```python
from build123d import *

# Parameters (mm, degrees)
F0_R      = 2.5
F1_DEPTH  = 85
F3_DEPTH  = 2.5
F5_DEPTH  = 25
F8_DEPTH  = 25
F9_DEPTH  = 25
F11_DEPTH = 25
F14_DEPTH = 102
F16_REACH = 96.5783545855
F18_REACH = 97.7333268634
F19_W     = 5
F19_H     = 41.5
F20_DEPTH = 25


with BuildPart() as f1:
    # F0 (on Front) → F1 (new body)
    with BuildSketch(Plane.XZ):
        Circle(F0_R)
    extrude(amount=F1_DEPTH)

    # F2 (on Right) → F3 (join, symmetric)
    with BuildSketch(Plane.YZ):
        Polygon((-69, 0), (-16, 0), (-22.4278760969, 7.6604444312), (-62.5721239031, 7.6604444312), align=None)
    extrude(amount=F3_DEPTH, both=True)

    # F4 (on face) → F5 (cut)
    with BuildSketch(Plane(origin=(-2.5, 0, 0), x_dir=(0, -1, 0), z_dir=(-1, 0, 0))):
        Polygon((56.5, 3), (53.5, 3), (50.5, 3), (44.1691353238, -4.5448307221), (62.8308646762, -4.5448307221), align=None)
        Polygon((40.8308646762, -4.5448307221), (34.5, 3), (31.5, 3), (28.5, 3), (22.1691353238, -4.5448307221), align=None)
    extrude(amount=-F5_DEPTH, mode=Mode.SUBTRACT)

    # F7 (on face) → F8 (cut)
    with BuildSketch(Plane(origin=(-2.5, 0, 0), x_dir=(0, -1, 0), z_dir=(-1, 0, 0))):
        Polygon((19.9172031134, 7.5), (22.2932472338, 7.5), (22.4278760969, 7.6604444312), (62.5721239031, 7.6604444312), (62.7067527662, 7.5), (66.5233954787, 7.5), (66.5233954787, 10.3880958632), (19.9172031134, 10.3880958632), align=None)
    extrude(amount=-F8_DEPTH, mode=Mode.SUBTRACT)

    # F6 (on face) → F9 (cut)
    with BuildSketch(Plane(origin=(0, 0, 3), x_dir=(1, 0, 0), z_dir=(0, 0, -1))):
        with BuildLine():
            ThreePointArc((1.45, 53.5), (1.0253048327, 54.5253048327), (0, 54.95))
            Line((0, 54.95), (0, 52.05))
            ThreePointArc((0, 52.05), (1.0253048327, 52.4746951673), (1.45, 53.5))
        make_face()
        with BuildLine():
            Line((0, 52.05), (0, 54.95))
            ThreePointArc((0, 54.95), (-1.45, 53.5), (0, 52.05))
        make_face()
    extrude(amount=-F9_DEPTH, mode=Mode.SUBTRACT)

    # F10 (on face) → F11 (cut)
    with BuildSketch(Plane(origin=(0, 0, 3), x_dir=(1, 0, 0), z_dir=(0, 0, -1))):
        with BuildLine():
            ThreePointArc((1.45, 31.5), (1.0253048327, 32.5253048327), (0, 32.95))
            Line((0, 32.95), (0, 30.05))
            ThreePointArc((0, 30.05), (1.0253048327, 30.4746951673), (1.45, 31.5))
        make_face()
        with BuildLine():
            Line((0, 30.05), (0, 32.95))
            ThreePointArc((0, 32.95), (-1.45, 31.5), (0, 30.05))
        make_face()
    extrude(amount=-F11_DEPTH, mode=Mode.SUBTRACT)

    # F13 (on face) → F14 (cut)
    with BuildSketch(Plane.XZ.offset(85)):
        with BuildLine():
            ThreePointArc((2.4, 0), (0, -2.4), (-2.4, 0))
            Line((-2.4, 0), (-2.4, 9.7710704431))
            Line((-2.4, 9.7710704431), (-6.1972029507, 9.7710704431))
            Line((-6.1972029507, 9.7710704431), (-6.1972029507, -5.7614380494))
            Line((-6.1972029507, -5.7614380494), (5.5722752586, -5.7614380494))
            Line((5.5722752586, -5.7614380494), (5.5722752586, 8.8547384366))
            Line((5.5722752586, 8.8547384366), (2.4, 9.1607915238))
            Line((2.4, 9.1607915238), (2.4, 0))
        make_face()
    extrude(amount=-F14_DEPTH, mode=Mode.SUBTRACT)

    f16_end = Plane(origin=(0, -64.9529870595, 4.8230422111), x_dir=(0, -0.6427876097, -0.7660444431), z_dir=(0, -0.7660444431, 0.6427876097))
    # F15 (on face) → F16 (cut, up to a plane its end follows)
    with BuildSketch(Plane.XZ.offset(85)):
        with BuildLine():
            ThreePointArc((-2.4, 0), (0, 2.4), (2.4, 0))
            Line((2.4, 0), (4.8319334164, 0))
            Line((4.8319334164, 0), (4.1808704846, 8.0774491653))
            Line((4.1808704846, 8.0774491653), (-2.9383567162, 8.0774491653))
            Line((-2.9383567162, 8.0774491653), (-3.4620375372, 0))
            Line((-3.4620375372, 0), (-2.4, 0))
        make_face()
    f16_long = extrude(amount=-F16_REACH, mode=Mode.PRIVATE)
    add(split(f16_long, bisect_by=f16_end, keep=Keep.TOP, mode=Mode.PRIVATE), mode=Mode.SUBTRACT)

    f18_end = Plane(origin=(0, -20.0470129405, 4.8230422111), x_dir=(0, -0.6427876097, 0.7660444431), z_dir=(0, 0.7660444431, 0.6427876097))
    # F17 (on face) → F18 (cut, up to a plane its end follows)
    with BuildSketch(Plane(origin=(0, 0, 0), x_dir=(-1, 0, 0), z_dir=(0, 1, 0))):
        with BuildLine():
            ThreePointArc((-2.4, 0), (0, 2.4), (2.4, 0))
            Line((2.4, 0), (3.9089121856, 0))
            Line((3.9089121856, 0), (4.3247276917, 8.6870230734))
            Line((4.3247276917, 8.6870230734), (-4.9837511033, 8.3660408854))
            Line((-4.9837511033, 8.3660408854), (-3.4170385916, 0))
            Line((-3.4170385916, 0), (-2.4, 0))
        make_face()
    f18_long = extrude(amount=-F18_REACH, mode=Mode.PRIVATE)
    add(split(f18_long, bisect_by=f18_end, keep=Keep.TOP, mode=Mode.PRIVATE), mode=Mode.SUBTRACT)

    # F19 (on face) → F20 (cut)
    with BuildSketch(Plane.YZ.offset(2.4)):
        Polygon((0, -4.5159468427), (0, -2.4), (0, 2.4), (-7, 2.4), (-7, -4.5159468427), align=None)
        with Locations((-82.5, 0)):
            Rectangle(F19_W, F19_H)
    extrude(amount=-F20_DEPTH, mode=Mode.SUBTRACT)


solid = f1.part
```
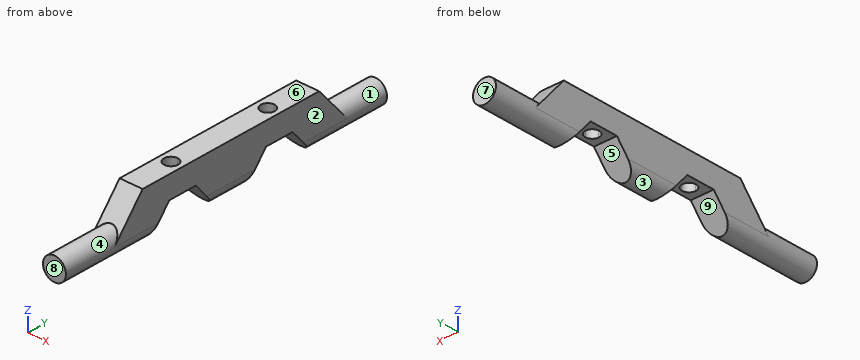
Model file for the job. Use its own axes, mm. Face numbers are marked on the shaded views. A direction names the side the tool comes from. Give positions to 0.01 mm unless a question says otherwise; leave off trailing zeros. Loops run counter-clockwise (first coordinate to the right, second up) from the corner with the lowest first, then second, coordinate; pieces in that order, holes last. Notation, with made-up numbers: (54.25, 0.25) - (68.25, 0.25) arc R24 ccw to (68.25, 32.25) - close; hole circle Ø7 at (76, 1). An arc over 180 degrees is marked (long way). One line per item, written item: value. Start each with the question number.
1. Pin check, flat tips, straight feed: pin 1 (1.5 mm diameter, centred on x = -2, y = -35.5, fed in from -Z); pin 2 (1.5 mm diameter, centred on y = -72.5, z = 2, fed in from -X); pin 3 (1.5 mm diameter, centred on x = 1.5, z = 6, fed in from +Y). Stop position of each tip, or through.
2. Slice it at B-B (z = 5.5). List the corners of the cut face in (x, y).
3. Probe L1, parallel to Y at x = -1.25, z = 4.5; L2, parallel to Y at x = -1.5, z = -1; L3, parallel to Z at x = 0.2, y = -70.5. List the from-to ranges inside material, lowest first. Write a range as from..to.
4. Slice it at C-C (y = -36). List the corners of the cut face in (x, z).
5. Slice it at A-A (z = -1.5). List the corners of the cut face in (x, y), plus the area to 3 significant figures.
6. Pull direction Y, two halves, no side cores. Call the marked faces 6, 7, 8 and 9: pulls with the +Y half, pulls with the -Y half, needs draft (parallel to the pull), parting line crosses it, or undercut.
7. Which spindle directions (+Z, -Z, +X, -X, +Y, -Y) get a long thin tool onto all of the face, cutting with end or side? Do the marked faces 1, 2, 3, 4 and 5. Say none if no direction does.
Solution:
1. pin 1: stops at z = 0.91
1. pin 2: stops at x = -2.05
1. pin 3: stops at y = -20.41
2. outline: (-2.4, -64.38) - (2.4, -64.38) - (2.4, -20.62) - (-2.4, -20.62) - close; hole circle Ø2.9 at (0, -53.5); hole circle Ø2.9 at (0, -31.5)
3. L1: y = -65.22..-54.23, -52.77..-32.23, -30.77..-19.78
3. L2: y = -80..-59.86, -47.14..-37.86, -25.14..-7
3. L3: z = -2.39..2.39
4. outline: (-2.4, 1.21) - (2.4, 1.21) - (2.4, 7.66) - (-2.4, 7.66) - close
5. outline: (-1.87, -80) - (1.87, -80) - (1.87, -60.28) - (-1.87, -60.28) - close; (-1.87, -46.72) - (1.87, -46.72) - (1.87, -38.28) - (-1.87, -38.28) - close; (-1.87, -24.72) - (1.87, -24.72) - (1.87, -7) - (-1.87, -7) - close
5. area: 172 mm^2
6. face 6: needs draft
6. face 7: pulls with the +Y half
6. face 8: pulls with the -Y half
6. face 9: undercut
7. face 1: +Y
7. face 2: +Z, -Z, +X, +Y, -Y
7. face 3: -Z, +Y, -Y
7. face 4: -Y
7. face 5: -Z, +X, -X
